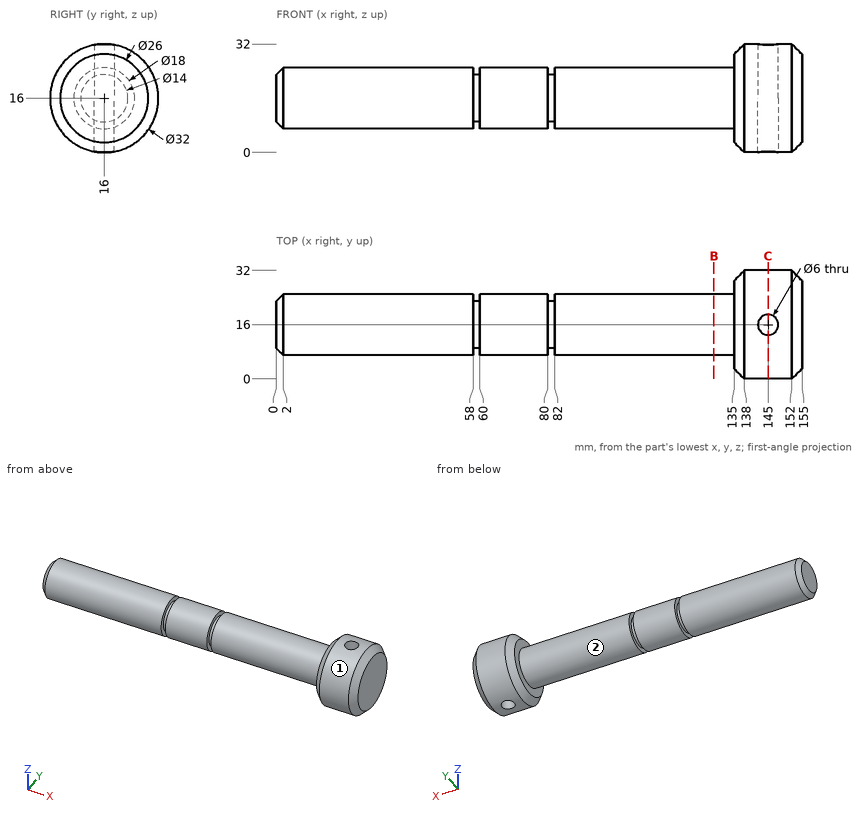
The figure shows three views and two pictorial views of one solid part (mm, origin at its lowest corner). Answer the questions. A direction names the side the tool comes from. Coordinates: 2 decimals unless noted, no trailing zeros. Order: outer loops, then holes, each group sorted by start corner. A loop starts at its lowest first (then second) coordinate and runs counter-clockwise, first axis right, second up.
Q1. Which of the six approach directions +Z, -Z, +X, -X, +Y, -Y give full straight-line access (tool end or side, diameter ignored) to the marked faces 1 and 2?
Q2. Given P1, Ø7, axis at x = 145, y = 16, coming from the -Z side; P2, Ø4, axis at x = 96.5, z = 16.5, coming from the -Y side; P3, Ø5, axis at x = 34, z = 23.5, coming from the -Y side; P4, Ø5, axis at x = 77.5, z = 8, coming from the -Y side, each flat-ended and moving along its own axis, determine where each tip first touches the part or whether it passes through.
Q3. A cutting plane is placed at C-C, the plane x = 145. Write down the section's boundary in (y, z).
Q4. Consider line 1 (X direction, y = 10, z = 9.5); line 2 (Y direction, x = 11, z = 16.5); line 3 (X direction, y = 24.5, z = 24.5). Determine where each line is inside the solid, lowest interval first.
Q5. A cutting plane is placed at B-B, the plane x = 129. Write down the section's boundary in (y, z).
Answers follow:
1. face 1: +X, -X
1. face 2: -X
2. P1: stops at z = 0
2. P2: stops at y = 7
2. P3: stops at y = 8.52
2. P4: stops at y = 8.88
3. outline: (13, 0.28) - (13, 31.72) arc R16 ccw to start; (19, 0.28) arc R16 ccw to (19, 31.72) - close
4. line 1: x = 1.85 to 58, 60 to 80, 82 to 155
4. line 2: y = 7.01 to 24.99
4. line 3: x = 135 to 155
5. outline: circle Ø18 at (16, 16)
